For this review, take the finished solid that the model builds, in its own axes (mm). A direction names the side the tool comes from. Round coordinates to 2 decimals unless told otherwise and drop trailing zeros. Order: outer loops, then holes, each group sorted by start corner. A loop starts at its lowest first (then second) coordinate and runs counter-clockwise, first axis right, second up. Notation, with made-up numbers: M 39.5,86.25 L 56.5,86.25 A17 ccw 56.5,104.25 Z; hole C -36.75,49 d2. An arc over 180 degrees is marked long. Use a Markdown table: item, result.
from build123d import *

# Parameters (mm, degrees)
F1_DEPTH = 63.5
F2_DEPTH = 25.4
F3_DEPTH = 7.9375
F0_W     = 25.4
F0_H     = 19.05
F4_DEPTH = 25.4
F6_R     = 6.35


with BuildPart() as f1:
    # F0 (on Front) → F1 (new body, symmetric)
    with BuildSketch(Plane.XZ):
        Polygon((-41.275, 9.525), (-41.275, -9.525), (41.275, -9.525), (41.275, 9.525), (22.225, 9.525), align=None)
    extrude(amount=F1_DEPTH, both=True)

    # F0 (on Front) → F2 (join, symmetric)
    with BuildSketch(Plane.XZ):
        with BuildLine():
            Line((22.225, 9.525), (41.275, 9.525))
            Line((41.275, 9.525), (41.275, 27.0002))
            ThreePointArc((41.275, 27.0002), (45.9246798487, 38.2255201513), (57.15, 42.8752))
            Line((57.15, 42.8752), (62.3217315116, 42.8752))
            Line((62.3217315116, 42.8752), (62.3217315116, 61.9252))
            Line((62.3217315116, 61.9252), (57.15, 61.9252))
            add(Edge.make_bspline(
                [(55.6203273588, 61.8916850158), (56.1294251185, 61.9058990464), (56.639326625, 61.9170854616), (57.15, 61.9252)],
                knots=[110.4319750844, 110.4319750844, 110.4319750844, 110.4319750844, 111.5045361635, 111.5045361635, 111.5045361635, 111.5045361635], degree=3))
            ThreePointArc((55.6203273588, 61.8916850158), (31.9192703039, 51.1490282118), (22.225, 27.0002))
            Line((22.225, 27.0002), (22.225, 9.525))
        make_face()
    extrude(amount=F2_DEPTH, both=True)

    # F0 (on Front) → F3 (join, symmetric)
    with BuildSketch(Plane.XZ):
        with BuildLine():
            add(Edge.make_bspline(
                [(-41.275, 9.525), (-40.6936184634, 26.8690425338), (3.2031063652, 60.4281940287), (55.6203273588, 61.8916850158)],
                knots=[0, 0, 0, 0, 110.4319750844, 110.4319750844, 110.4319750844, 110.4319750844], degree=3))
            Line((-41.275, 9.525), (22.225, 9.525))
            Line((22.225, 9.525), (22.225, 27.0002))
            ThreePointArc((22.225, 27.0002), (31.9192703039, 51.1490282118), (55.6203273588, 61.8916850158))
        make_face()
    extrude(amount=F3_DEPTH, both=True)

    # F0 (on Front) → F4 (join, symmetric)
    with BuildSketch(Plane.XZ):
        with Locations((75.0217315116, 52.4002)):
            Rectangle(F0_W, F0_H)
    extrude(amount=F4_DEPTH, both=True)

    # F0 (on Front) → F5 (revolve)
    with BuildSketch(Plane.XZ):
        Polygon((87.7217315116, 66.675), (87.7217315116, 61.9252), (87.7217315116, 42.8752), (87.7217315116, 38.1), (113.1217315116, 38.1), (113.1217315116, 66.675), align=None)
    revolve(axis=Axis((87.7217315116, 0, 52.3875), (0, 0, 1)))

    # F6
    f6_edges = [f1.edges().sort_by_distance(p)[0] for p in [
        (41.275, 63.5, 0),
        (-41.275, 63.5, 0),
        (-41.275, -63.5, 0),
        (41.275, -63.5, 0),
    ]]
    fillet(f6_edges, radius=F6_R)


solid = f1.part
Q1. Wall thickness on line 1 along X through (y, z) = (-47, -4.5) (3 decimals); line 2 along Z through (x, y) = (-25.5, 19) (3 decimals); line 3 along Z through (x, y) = (101, -13.5) (3 decimals): over which ranges is each line inside the solid? List them lowest first. Write a range as [from, to].
Determined:
| item | result |
|---|---|
| line 1 | x = [-41.275, 41.275] |
| line 2 | z = [-9.525, 9.525] |
| line 3 | z = [38.1, 66.675] |
Q2. Clearance check with flat-ended pins moving along their axes: pin 1 (1.5 mm diameter, centred on x = 80.5, z = 49, fed in from +Y); pin 2 (15.5 mm diameter, centred on x = -13, z = 30.5, fed in from +Y); pin 3 (11 mm diameter, centred on y = 26, z = 0, fed in from +X) (3 decimals). State where each tip first meets the part, or that it passes through.
Determined:
| item | result |
|---|---|
| pin 1 | stops at y = 25.4 |
| pin 2 | stops at y = 7.94 |
| pin 3 | stops at x = 41.275 |
Q3. Add section A-A (z = -3). Write out the cut boundary in (x, y) (3 decimals), then the cut area to 3 significant figures.
Determined:
| item | result |
|---|---|
| outline | M -41.275,-57.15 A6.35 ccw -34.925,-63.5 L 34.925,-63.5 A6.35 ccw 41.275,-57.15 L 41.275,57.15 A6.35 ccw 34.925,63.5 L -34.925,63.5 A6.35 ccw -41.275,57.15 Z |
| area | 10,400 mm^2 |
Q4. Machinability: for faces 1 (the flat face through (22.225, -17, 18)), 2 (the flat face through (22.225, 17, 18)), 3 (the cylindrical face through (45.8, -0.4, 38.1)), which of the approach directions +Z, -Z, +X, -X, +Y, -Y give a long, thin tool a straight path to every point of the face, cutting with its end or side? Answer none if there is none.
Determined:
| item | result |
|---|---|
| face 1 | +Z, -X, -Y |
| face 2 | +Z, -X, +Y |
| face 3 | -Z, +Y, -Y |
Q5. Add section B-B (x = 72.5). Write out the cut boundary in (y, z) (3 decimals).
Determined:
| item | result |
|---|---|
| outline | M -25.4,42.875 L -20.334,42.875 L -20.334,38.1 L 20.334,38.1 L 20.334,42.875 L 25.4,42.875 L 25.4,61.925 L 20.334,61.925 L 20.334,66.675 L -20.334,66.675 L -20.334,61.925 L -25.4,61.925 Z |
Q6. Add section C-C (y = -40.5). Write out the cut boundary in (x, z) (3 decimals), then the cut area to 3 significant figures.
Determined:
| item | result |
|---|---|
| outline | M -41.275,-9.525 L 41.275,-9.525 L 41.275,9.525 L -41.275,9.525 Z |
| area | 1,570 mm^2 |
